```python
from build123d import *

# Parameters (mm, degrees)
BOSS_EXTRU_1_DEPTH = 1.5
BOSS_EXTRU_2_DEPTH = 11


with BuildPart() as part:
    # Esquisse1 → Boss.-Extru.1 (new body)
    with BuildSketch(Plane.XY):
        with BuildLine():
            Line((-11, 10), (11, 10))
            Line((11, 10), (11, -14))
            Line((11, -14), (33.226495452, -14))
            ThreePointArc((33.226495452, -14), (35, -25), (33.226495452, -36))
            Line((33.226495452, -36), (11, -36))
            Line((11, -36), (11, -60))
            Line((11, -60), (-11, -60))
            Line((-11, -60), (-11, -36))
            Line((-11, -36), (-33.226495452, -36))
            ThreePointArc((-33.226495452, -36), (-35, -25), (-33.226495452, -14))
            Line((-33.226495452, -14), (-11, -14))
            Line((-11, -14), (-11, 10))
        make_face()
        with BuildLine():
            Line((1.5, 5), (1.5, -11))
            ThreePointArc((1.5, -11), (0, -12.5), (-1.5, -11))
            Line((-1.5, -11), (-1.5, 5))
            ThreePointArc((-1.5, 5), (0, 6.5), (1.5, 5))
        make_face(mode=Mode.SUBTRACT)
        with BuildLine():
            Line((1.5, -39), (1.5, -55))
            ThreePointArc((1.5, -55), (0, -56.5), (-1.5, -55))
            Line((-1.5, -55), (-1.5, -39))
            ThreePointArc((-1.5, -39), (0, -37.5), (1.5, -39))
        make_face(mode=Mode.SUBTRACT)
    extrude(amount=BOSS_EXTRU_1_DEPTH)

    # Esquisse3 → Boss.-Extru.2 (add)
    with BuildSketch(Plane.XY.offset(1.5)):
        Polygon((28.544164415, -33.139950571), (32.392821374, -29.291293612), (30.12954231, -27.028014548), (26.280885351, -30.876671507), align=None)
    extrude(amount=BOSS_EXTRU_2_DEPTH)


solid = part.part
```
Model file for the job. Use its own axes, mm. A direction names the side the tool comes from. Give positions to 0.01 mm unless a question says otherwise; leave off trailing zeros. Order: outer loops, then holes, each group sorted by start corner. A loop starts at its lowest first (then second) coordinate and runs counter-clockwise, first axis right, second up.
1) Wall check: probe 1 along X at (y, z) = (0, 1.25); probe 2 along Z at (x, y) = (7, -46); probe 3 along Y at (x, z) = (28, 6.5). Give the ranges that are in metal, low to high.
2) Mould opens along X. For faces 4 (the flat face through (0, -25, 1.5)), 5 (the cylindrical face through (0, 6.5, 0.7)), 6 (the flat face through (31.3, -28.2, 6.9)) say: +X half, -X half, draft (parallel to the pull), parting line (faces both ways), or undercut.
3) Pin check, flat tips, straight feed: pin 1 (1.6 mm diameter, centred on y = -2, z = 1, fed in from +X); pin 2 (1.6 mm diameter, centred on y = -49.5, z = 1, fed in from -X); pin 3 (1.6 mm diameter, centred on x = 23.5, z = 0.5, fed in from +Y); pin 4 (10 mm diameter, centred on x = 17.5, y = 1.5, fed in from -Z). Stop position of each tip, or through.
4) Saw through at B-B, the plane y = -42. Write the cut outline in (x, z), then the cut area to 3 significant figures.
5) Saw through at A-A, the plane x = 0. Write the cut outline in (y, z), then the cut area to 3 significant figures.
6) Saw through at D-D, the plane x = 24. Write the cut outline in (y, z), then the cut area to 3 significant figures.
7) Saw through at C-C, the plane z = 7. Write the cut outline in (x, y).
8) 3-axis set-ups, long thin cutter, end or side, ignore diameter. For faces 1 (the cylindrical face through (0, -37.5, 0.7)), 2 (the flat face through (11, -2, 1)), 3 (the flat face through (-11, -2, 1)): which of +Z, -Z, +X, -X, +Y, -Y reach the whole face in a straight line?
Computed:
1. probe 1: x = -11 to -1.5, 1.5 to 11
1. probe 2: z = 0 to 1.5
1. probe 3: y = -32.6 to -29.16
2. face 4: draft
2. face 5: undercut
2. face 6: +X half
3. pin 1: stops at x = 11
3. pin 2: stops at x = -11
3. pin 3: stops at y = -14
3. pin 4: passes through
4. outline: (-11, 0) - (-1.5, 0) - (-1.5, 1.5) - (-11, 1.5) - close; (1.5, 0) - (11, 0) - (11, 1.5) - (1.5, 1.5) - close
4. area: 28.5 mm2
5. outline: (-60, 0) - (-56.5, 0) - (-56.5, 1.5) - (-60, 1.5) - close; (-37.5, 0) - (-12.5, 0) - (-12.5, 1.5) - (-37.5, 1.5) - close; (6.5, 0) - (10, 0) - (10, 1.5) - (6.5, 1.5) - close
5. area: 48.0 mm2
6. outline: (-36, 0) - (-14, 0) - (-14, 1.5) - (-36, 1.5) - close
6. area: 33.0 mm2
7. outline: (26.28, -30.88) - (28.54, -33.14) - (32.39, -29.29) - (30.13, -27.03) - close
8. face 1: +Z, -Z
8. face 2: +Z, -Z, +X, +Y
8. face 3: +Z, -Z, -X, +Y
